```python
from build123d import *

# Parameters (mm, degrees)
F0_R     = 1.85
F1_DEPTH = 0.95
F2_W     = 4.5
F2_H     = 4.2
F3_DEPTH = 3.25
F4_R     = 2.09999
F5_R     = 1.15
F6_DEPTH = 25


# Not quite as in the source:
# - a fillet or chamfer is up to 0.001 mm smaller than in the source, because OpenCascade refuses the exact size


with BuildPart() as f1:
    # F0 (on Top) → F1 (new body)
    with BuildSketch(Plane.XY):
        with BuildLine():
            Line((10.9, 1.2), (15.4, 1.2))
            Line((15.4, 1.2), (15.4, 5.4))
            Line((15.4, 5.4), (10.9, 5.4))
            Line((10.9, 5.4), (10.2120730928, 5.4))
            ThreePointArc((10.2120730928, 5.4), (9.9013861494, 5.4146577616), (9.5934591909, 5.4585008344))
            Line((9.5934591909, 5.4585008344), (3.9186139019, 6.5414991656))
            ThreePointArc((3.9186139019, 6.5414991656), (3.6106869434, 6.5853422384), (3.3, 6.6))
            ThreePointArc((3.3, 6.6), (0.9665476221, 5.6334523779), (0, 3.3))
            ThreePointArc((0, 3.3), (0.9665476221, 0.9665476221), (3.3, 0))
            ThreePointArc((3.3, 0), (3.6106869434, 0.0146577616), (3.9186139019, 0.0585008344))
            Line((3.9186139019, 0.0585008344), (9.5934591909, 1.1414991656))
            ThreePointArc((9.5934591909, 1.1414991656), (9.9013861494, 1.1853422384), (10.2120730928, 1.2))
            Line((10.2120730928, 1.2), (10.9, 1.2))
        make_face()
        with Locations((3.3, 3.3)):
            Circle(F0_R, mode=Mode.SUBTRACT)
    extrude(amount=F1_DEPTH)

    # F2 (on face) → F3 (join)
    with BuildSketch(Plane.XY.offset(0.95)):
        with Locations((13.15, 3.3)):
            Rectangle(F2_W, F2_H)
    extrude(amount=F3_DEPTH)

    # F4 (radius 2.1 in the source; OpenCascade refuses exactly that, so slightly less here)
    f4_edges = [f1.edges().sort_by_distance(p)[0] for p in [
        (13.15, 5.4, 4.2),
        (13.15, 1.2, 4.2),
    ]]
    fillet(f4_edges, radius=F4_R)

    # F5 (on face) → F6 (cut)
    with BuildSketch(Plane.YZ.offset(15.4)):
        with Locations((3.3, 2.1)):
            Circle(F5_R)
    extrude(amount=-F6_DEPTH, mode=Mode.SUBTRACT)


solid = f1.part
```
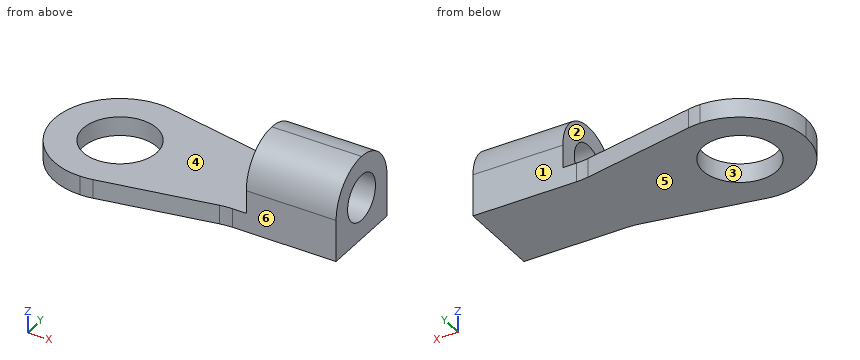
Build history of the part. All positions in model axes, mm. Face numbers are marked on the shaded views. A direction names the side the tool comes from. Coordinates: 2 decimals unless noted, no trailing zeros. Write each loop counter-clockwise with the first axis right and the second up, starting at its lowest first coordinate (ties: lowest second). Pieces come first, ordered by that corner, then holes.
1. Pull direction X, two halves, no side cores. Call the marked faces 1, 2 and 3: released by +X, released by -X, zero draft, split by the parting line, or undercut.
Answer block:
face 1: zero draft
face 2: released by -X
face 3: undercut
2. Band-saw the part on B-B, the plane z = 1.95. Give the cut face in (x, y), and give its area (3 significant figures).
Answer block:
outline: (10.9, 1.2) - (15.4, 1.2) - (15.4, 2.16) - (10.9, 2.16) - close; (10.9, 4.44) - (15.4, 4.44) - (15.4, 5.4) - (10.9, 5.4) - close
area: 8.64 mm2
3. Band-saw the part on C-C, the plane x = 10.75. Give the cut face in (y, z), and give its area (3 significant figures).
Answer block:
outline: (1.2, 0) - (5.4, 0) - (5.4, 0.95) - (1.2, 0.95) - close
area: 3.99 mm2
4. 3-axis set-ups, long thin cutter, end or side, ignore diameter. For the marked faces 4, 5 and 6: which of +Z, -Z, +X, -X, +Y, -Y reach the whole face in a straight line?
Answer block:
face 4: +Z, -X, +Y, -Y
face 5: -Z, +X, -X, +Y, -Y
face 6: +Z, -Z, +X, -Y
5. Band-saw the part on A-A, the plane y = 1.75. Give the cut face in (x, z), and give its area (3 significant figures).
Answer block:
outline: (0.39, 0) - (2.29, 0) - (2.29, 0.95) - (0.39, 0.95) - close; (4.31, 0) - (15.4, 0) - (15.4, 3.52) - (10.9, 3.52) - (10.9, 0.95) - (4.31, 0.95) - close
area: 23.9 mm2
6. Band-saw the part on D-D, the plane y = 1. Give the cut face in (x, z), and give its area (3 significant figures).
Answer block:
outline: (0.93, 0) - (8.85, 0) - (8.85, 0.95) - (0.93, 0.95) - close
area: 7.52 mm2
7. Drill centre lines: probe 1 along Z at (x, y) = (12.1, 3.3); probe 2 along X at (y, z) = (3.25, 0.35); probe 3 along Z at (x, y) = (10, 1.5). Where is each one in solid material? Low to high.
Answer block:
probe 1: z = 0 to 0.95, 3.25 to 4.2
probe 2: x = 0 to 1.45, 5.15 to 15.4
probe 3: z = 0 to 0.95
8. Drop flat-ended pins along their axis: pin 1 (1.7 mm diameter, centred on x = 12.5, z = 1.5, fed in from -Y); pin 2 (0.6 mm diameter, centred on x = 12, z = 1.5, fed in from +Y); pin 3 (1.5 mm diameter, centred on x = 2, z = 3.5, fed in from -Y). Give the stop position or say it passes through.
Answer block:
pin 1: stops at y = 1.2
pin 2: stops at y = 5.4
pin 3: passes through
